Source: CAD feature listing. Evaluate the final solid. Frame: model axes, mm. Face numbers are marked on the shaded views. Coordinates: 2 decimals unless noted, no trailing zeros. Write each loop counter-clockwise with the first axis right and the second up, starting at its lowest first coordinate (ties: lowest second). Pieces come first, ordered by that corner, then holes. Notation, with made-up numbers: M -39,54 L -20,54 A19 ccw -20,60 Z; hole C -25.5,-28.75 d1. An arc over 180 degrees is marked long. Answer as CSV lines item,"result". Start each with the question number.
1. Line query: probe 1 along X at (y, z) = (-6.5, 18); probe 2 along Z at (x, y) = (-11, -20); probe 3 along Z at (x, y) = (71, -5). Output: solid intervals per line, ascending. Write a range as [from, to].
2. Section D-D on y = -16. Return the cut outline in (x, z).
3. Section C-C on y = -28. Return the cut outline in (x, z), plus the area to 3 significant figures.
4. Contact query for flat-ended pins moving along their axis: pin 1 Ø8 at (x, z) = (53, 15.5) entering from -Y (3 decimals); pin 2 Ø10 at (x, y) = (-53.5, 20.5) entering from +Z; pin 3 Ø3 at (x, y) = (73, -3.5) entering from +Z. Output: stop coordinate, or through.
5. Section B-B on z = 19.25. Return the cut outline in (x, y), plus the area to 3 significant figures.
6. Section A-A on x = 12. Return the cut outline in (y, z) (3 decimals), plus the area to 3 significant figures.
7. Mould query, pull axis X, two halves, no side actions, for the marked faces 1, 2, 3 and 4. Classes: pulls with the +X half, pulls with the -X half, needs draft (parallel to the pull), parting line crosses it, or undercut.
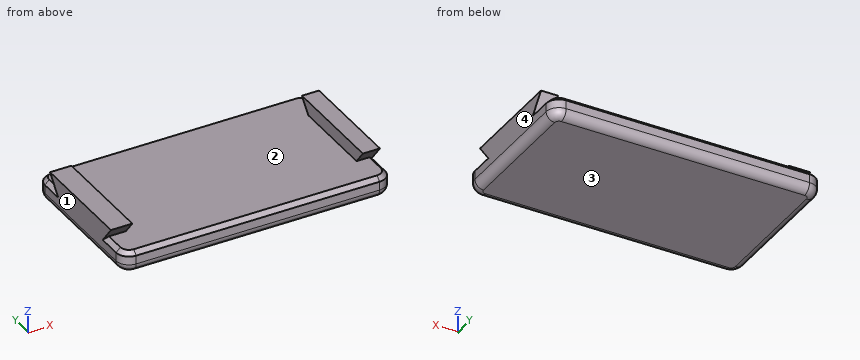
```python
from build123d import *

# Parameters (mm, degrees)
F0_W      = 149.86
F0_H      = 80.01
F1_DEPTH  = 12.7
F0_W_2    = 160.02
F0_H_2    = 90.17
F2_DEPTH  = 12.7
F3_R      = 7.62
F4_R      = 5.08
F7_W      = 50.8
F7_H      = 6.35
F8_DEPTH  = 12.7
F9_W      = 50.8
F9_H      = 6.35
F10_DEPTH = 10.16
F11_SIZE  = 2.54


# Not quite as in the source:
# - a feature names something its author has since deleted; it is built from what else it names


with BuildPart() as f1:
    # F0 (on Top) → F1 (new body)
    with BuildSketch(Plane.XY):
        Rectangle(F0_W, F0_H)
    extrude(amount=F1_DEPTH)

    # F0 (on Top) → F2 (join)
    with BuildSketch(Plane.XY):
        Rectangle(F0_W_2, F0_H_2)
        Rectangle(F0_W, F0_H, mode=Mode.SUBTRACT)
    extrude(amount=F2_DEPTH)

    # F3
    f3_edges = [f1.edges().sort_by_distance(p)[0] for p in [
        (-80.01, 45.085, 6.35),
        (-80.01, -45.085, 6.35),
        (80.01, -45.085, 6.35),
        (80.01, 45.085, 6.35),
    ]]
    fillet(f3_edges, radius=F3_R)

    # F4
    f4_edges = [f1.edges().sort_by_distance(p)[0] for p in [
        (-80.01, 0, 0),
        (0, 45.085, 0),
        (80.01, 0, 0),
        (77.778154, 42.853154, 0),
        (77.778154, -42.853154, 0),
        (-77.778154, -42.853154, 0),
        (0, -45.085, 0),
        (-77.778154, 42.853154, 0),
    ]]
    fillet(f4_edges, radius=F4_R)

    # F7 (on face) → F8 (join)
    with BuildSketch(Plane.YZ.offset(-80.01)):
        Polygon((32.0707530211, 21.0250992866), (-32.0642467673, 21.0303084591), (-25.4, 12.7), (-25.4, 19.05), (25.4, 19.05), (25.4, 12.7), align=None)
        with Locations((0, 15.875)):
            Rectangle(F7_W, F7_H)
    extrude(amount=F8_DEPTH)

    # F9 (on face) → F10 (join)
    with BuildSketch(Plane.YZ.offset(80.01)):
        Polygon((32.0707530211, 21.0250992866), (-32.0642467673, 21.0303084591), (-25.4, 12.7), (-25.4, 19.05), (25.4, 19.05), (25.4, 12.7), align=None)
        with Locations((0, 15.875)):
            Rectangle(F9_W, F9_H)
    extrude(amount=-F10_DEPTH)

    # F11
    f11_edges = [f1.edges().sort_by_distance(p)[0] for p in [
        (0, 45.085, 12.7),
        (0, -45.085, 12.7),
        (-80.01, 31.4325, 12.7),
        (-80.01, -31.4325, 12.7),
        (-77.778154, 42.853154, 12.7),
        (-77.778154, -42.853154, 12.7),
        (77.778154, 42.853154, 12.7),
        (77.778154, -42.853154, 12.7),
        (80.01, -31.4325, 12.7),
        (80.01, 31.4325, 12.7),
    ]]
    chamfer(f11_edges, length=F11_SIZE)


solid = f1.part
```
Values:
1,probe 1,"[-80.01, -67.31], [69.85, 80.01]"
1,probe 2,"[0, 12.7]"
1,probe 3,"[0, 21.03]"
2,outline,"M -80.01,5.08 A5.08 ccw -74.93,0 L 74.93,0 A5.08 ccw 80.01,5.08 L 80.01,21.03 L 69.85,21.03 L 69.85,12.7 L -67.31,12.7 L -67.31,21.03 L -80.01,21.03 Z"
3,outline,"M -80.01,5.08 A5.08 ccw -74.93,0 L 74.93,0 A5.08 ccw 80.01,5.08 L 80.01,10.16 L 77.47,12.7 L -77.47,12.7 L -80.01,10.16 Z; M -80.01,15.95 L -67.31,15.95 L -67.31,21.03 L -80.01,21.03 Z; M 69.85,15.95 L 80.01,15.95 L 80.01,21.03 L 69.85,21.03 Z"
3,area,"2,130 mm²"
4,pin 1,"y = -43.745"
4,pin 2,"z = 12.7"
4,pin 3,"z = 21.03"
5,outline,"M -80.01,-30.64 L -67.31,-30.64 L -67.31,30.65 L -80.01,30.65 Z; M 69.85,-30.64 L 80.01,-30.64 L 80.01,30.65 L 69.85,30.65 Z"
5,area,"1,400 mm²"
6,outline,"M -45.085,5.08 A5.08 ccw -40.005,0 L 40.005,0 A5.08 ccw 45.085,5.08 L 45.085,10.16 L 42.545,12.7 L -42.545,12.7 L -45.085,10.16 Z"
6,area,"1,130 mm²"
7,face 1,"pulls with the -X half"
7,face 2,"undercut"
7,face 3,"needs draft"
7,face 4,"pulls with the +X half"
